from build123d import *

# Parameters (mm, degrees)
SKETCH2_R                = 60
SKETCH2_R_2              = 12.5
BOSS_EXTRUDE1_DEPTH      = 20
SKETCH3_R                = 42.5
CUT_EXTRUDE1_DEPTH       = 10
SKETCH4_R                = 6
CUT_EXTRUDE2_DEPTH       = 91
CIRPATTERN2_COUNT        = 5
BOSS_EXTRUDE3_DEPTH      = 2
BOSS_EXTRUDE3_DEPTH_BACK = 7
SKETCH6_R                = 13.5
SKETCH6_R_2              = 12.5


with BuildPart() as part:
    # Sketch2 → Boss-Extrude1 (new, symmetric)
    with BuildSketch(Plane.XY):
        Circle(SKETCH2_R)
        Circle(SKETCH2_R_2, mode=Mode.SUBTRACT)
    extrude(amount=BOSS_EXTRUDE1_DEPTH, both=True)

    # Sketch3 → Cut-Extrude1 (cut)
    with BuildSketch(Plane.XY.offset(20)):
        Circle(SKETCH3_R)
    cut_extrude1 = extrude(amount=-CUT_EXTRUDE1_DEPTH, mode=Mode.SUBTRACT)

    # Mirror2: Cut-Extrude1 across plane
    add(cut_extrude1.mirror(Plane.XY), mode=Mode.SUBTRACT)

    # Sketch4 → Cut-Extrude2 (cut, symmetric)
    with BuildSketch(Plane.XY.offset(10)):
        with Locations((0, 25)):
            Circle(SKETCH4_R)
    cut_extrude2 = extrude(amount=CUT_EXTRUDE2_DEPTH, both=True, mode=Mode.SUBTRACT)

    # CirPattern2: Cut-Extrude2 ×5 about axis
    cirpattern2_axis = Axis((0, 0, 0), (0, 0, 1))
    for i in range(1, CIRPATTERN2_COUNT):
        add(cut_extrude2.rotate(cirpattern2_axis, i * 360 / CIRPATTERN2_COUNT), mode=Mode.SUBTRACT)

    # Sketch5 → Cut-Revolve1 (revolve, cut)
    with BuildSketch(Plane(origin=(0, 0, 0), x_dir=(1, 0, 0), z_dir=(0, 1, 0))):
        Polygon((54, 13.535898385), (60, 17), (60, -17), (54, -13.535898385), align=None)
    revolve(axis=Axis((0, 0, 0), (0, 0, -1)), mode=Mode.SUBTRACT)

    # Sketch6 → Boss-Extrude3 (add, two sides: drawn at the far end of the back side and taken through both)
    with BuildSketch(Plane.XY.offset(10).offset(-BOSS_EXTRUDE3_DEPTH_BACK)):
        Circle(SKETCH6_R)
        with Locations(Location((0, 0, 0), (0, 0, 180))):
            Circle(SKETCH6_R_2, mode=Mode.SUBTRACT)
    extrude(amount=BOSS_EXTRUDE3_DEPTH + BOSS_EXTRUDE3_DEPTH_BACK)


solid = part.part
Read the model definition and answer for the solid it produces. Units are mm, in the model's axes. A direction names the side the tool comes from. Round coordinates to 2 decimals unless told otherwise and drop trailing zeros. Write each loop counter-clockwise with the first axis right and the second up, starting at its lowest first coordinate (ties: lowest second). Pieces come first, ordered by that corner, then holes.
Q1. Flat-ended cylindrical pins translate along their axes: P1, Ø4, axis at x = 31.5, z = 13, coming from the -Y side; P2, Ø1, axis at x = 5, z = 0, coming from the +Y side; P3, Ø4, axis at x = 16, z = 9.5, coming from the +Y side; P4, Ø11, axis at x = 0, y = 25, coming from the +Z side. Find the tip coordinate at first contact, or state that the pin passes through.
Values:
P1: stops at y = -47.15
P2: stops at y = 53.81
P3: stops at y = 52.15
P4: passes through
Q2. Straight lines are drawn through the part: line 1 (Y direction, x = -1, z = 12.5); line 2 (Y direction, x = 0, z = -1); line 3 (Y direction, x = 9.5, z = 2). For each, find the intervals that lie inside material, in ascending order.
Values:
line 1: y = -53.99 to -42.49, 42.49 to 53.99
line 2: y = -54 to -12.5, 12.5 to 19, 31 to 54
line 3: y = -53.16 to -23.23, -17.22 to -8.12, 8.12 to 53.16
Q3. Find section A-A on x = 0. State how many separate pieces and enclosed holes the cut face has, and give its area (3 significant figures).
Values:
separate pieces: 3
enclosed holes: 0
area: 2,000 mm2
Q4. A tool of negligible diameter and unlimited length cuts with its end or side. For faces 1 (the face through (9, -9, -10)), 2 (the face through (9, -9, 12)), 3 (the face through (-11.706, 52.716, -0.19)), 4 (the face through (-1.301, 19.143, 0.14)), from which of +Z, -Z, +X, -X, +Y, -Y can it reach the whole face along a straight path? Write none if from no direction.
Values:
face 1: -Z
face 2: +Z
face 3: none
face 4: +Z, -Z
Q5. Find section B-B on y = 0. Determine the outline of the cut face in (x, z), and give its area (3 significant figures).
Values:
outline: (-60, -20) - (-42.5, -20) - (-42.5, -10) - (-12.5, -10) - (-12.5, 12) - (-13.5, 12) - (-13.5, 10) - (-42.5, 10) - (-42.5, 20) - (-60, 20) - (-60, 17) - (-54, 13.54) - (-54, -13.54) - (-60, -17) - close; (12.5, -10) - (42.5, -10) - (42.5, -20) - (60, -20) - (60, -17) - (54, -13.54) - (54, 13.54) - (60, 17) - (60, 20) - (42.5, 20) - (42.5, 10) - (13.5, 10) - (13.5, 12) - (12.5, 12) - close
area: 2,240 mm2
Q6. Find section C-C on z = -6. Determine the outline of the cut face in (x, y).
Values:
outline: circle Ø108 at (0, 0); hole circle Ø12 at (-23.78, 7.73); hole circle Ø12 at (-14.69, -20.23); hole circle Ø25 at (0, 0); hole circle Ø12 at (0, 25); hole circle Ø12 at (14.69, -20.23); hole circle Ø12 at (23.78, 7.73)
Q7. The mould has two halves that part along X. Classify faces 5 (the face through (51.78, -16.31, 13.7)), 6 (the face through (0.824, 12.473, 0.846)), 7 (the face through (12, 41, 20)): released by +X, released by -X, zero draft, split by the parting line, or undercut.
Values:
face 5: split by the parting line
face 6: undercut
face 7: zero draft
